Geometry: see drawing. Coordinates: mm, zero at the bounding-box minimum. Round coordinates to 2 decimals unless told otherwise and drop trailing zeros. Write each loop counter-clockwise with the first axis right and the second up, starting at its lowest first coordinate (ties: lowest second). Pieces come first, ordered by that corner, then holes.
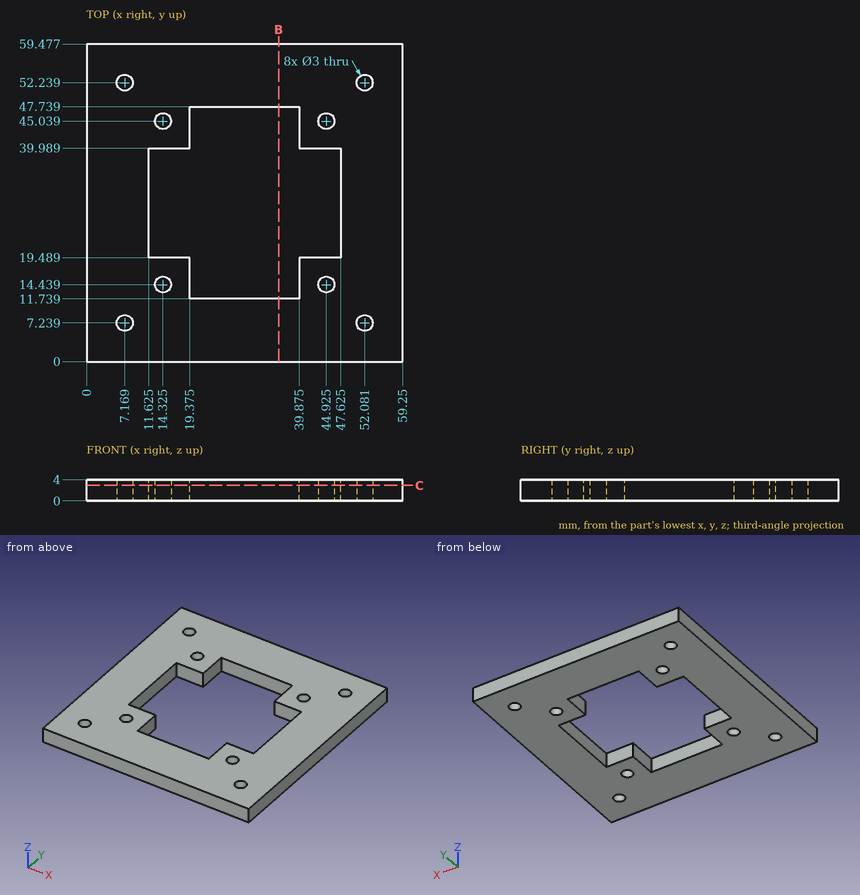
1) Material intervals for line 1 (Y direction, x = 32, z = 0.8); line 2 (Y direction, x = 41, z = 2.95); line 3 (Y direction, x = 7.5, z = 3.1) (1 decimal), sorted ascending.
Taken from the geometry:
line 1: y = 0 to 11.74, 47.74 to 59.48
line 2: y = 0 to 19.49, 39.99 to 59.48
line 3: y = 0 to 5.8, 8.7 to 50.8, 53.7 to 59.5
2) Section query C-C on z = 2.9. State how many separate pieces and enclosed holes the cut face has, then the cut area to 3 significant figures.
Taken from the geometry:
separate pieces: 1
enclosed holes: 9
area: 2,410 mm2
3) Contact query for a flat-ended pin moving along its axis: P1, Ø8, axis at x = 35.5, y = 20.5, coming from the -Z side. Output: stop coordinate, or through.
Taken from the geometry:
P1: passes through
4) Section query B-B on x = 36. Return the cut outline in (y, z).
Taken from the geometry:
outline: (0, 0) - (11.74, 0) - (11.74, 4) - (0, 4) - close; (47.74, 0) - (59.48, 0) - (59.48, 4) - (47.74, 4) - close
